from build123d import *

# Parameters (mm, degrees)
SKETCH2_W           = 52
SKETCH2_H           = 52
BOSS_EXTRUDE1_DEPTH = 70
SKETCH3_R           = 15
BOSS_EXTRUDE2_DEPTH = 20
SKETCH4_R           = 1
CUT_EXTRUDE1_DEPTH  = 5
SKETCH5_R           = 25
BOSS_EXTRUDE3_DEPTH = 8


with BuildPart() as part:
    # Sketch2 → Boss-Extrude1 (new body)
    with BuildSketch(Plane.XY):
        Rectangle(SKETCH2_W, SKETCH2_H)
    extrude(amount=BOSS_EXTRUDE1_DEPTH)

    # Sketch3 → Boss-Extrude2 (add)
    with BuildSketch(Plane.XY.offset(70)):
        Circle(SKETCH3_R)
    extrude(amount=BOSS_EXTRUDE2_DEPTH)

    # Sketch4 → Cut-Extrude1 (cut)
    with BuildSketch(Plane.XZ.offset(26)):
        with Locations((-16.5, 62)):
            Circle(SKETCH4_R)
        with Locations((-16.5, 28.5)):
            Circle(SKETCH4_R)
        with Locations((-1.5, 62)):
            Circle(SKETCH4_R)
        with Locations((-1.5, 28.5)):
            Circle(SKETCH4_R)
        with Locations((-1.5, 7)):
            Circle(SKETCH4_R)
        with Locations((-16.5, 7)):
            Circle(SKETCH4_R)
    extrude(amount=-CUT_EXTRUDE1_DEPTH, mode=Mode.SUBTRACT)

    # Sketch5 → Boss-Extrude3 (add)
    with BuildSketch(Plane.XY.offset(90)):
        Circle(SKETCH5_R)
    extrude(amount=-BOSS_EXTRUDE3_DEPTH)


solid = part.part
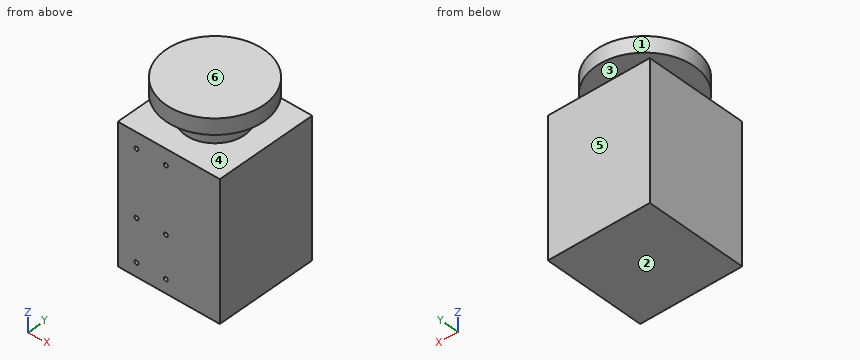
Verification items for the finished model (mm, model axes). Face numbers are marked on the shaded views. A direction names the side the tool comes from. Coordinates: 2 decimals unless noted, no trailing zeros. Order: outer loops, then holes, each group sorted by start corner. A loop starts at its lowest first (then second) coordinate and runs counter-clockwise, first axis right, second up.
Item 1: Section check D-D, the plane x = -1.5. Enter the section's corners in (y, z), then the cut area to 3 significant figures.
Filled in:
outline: (-26, 0) - (26, 0) - (26, 70) - (14.92, 70) - (14.92, 82) - (24.95, 82) - (24.95, 90) - (-24.95, 90) - (-24.95, 82) - (-14.92, 82) - (-14.92, 70) - (-26, 70) - (-26, 63) - (-21, 63) - (-21, 61) - (-26, 61) - (-26, 29.5) - (-21, 29.5) - (-21, 27.5) - (-26, 27.5) - (-26, 8) - (-21, 8) - (-21, 6) - (-26, 6) - close
area: 4,370 mm2
Item 2: Section check C-C, the plane y = -19.5. Enter the section's corners in (x, z).
Filled in:
outline: (-26, 0) - (26, 0) - (26, 70) - (-26, 70) - close; (-15.64, 82) - (15.64, 82) - (15.64, 90) - (-15.64, 90) - close
Item 3: Depth check by flat-ended pin: pin 1 (1.2 mm diameter, centred on x = -16.5, z = 28.5, fed in from -Y). Enter the tip coordinate at first touch or a pass-through.
Filled in:
pin 1: stops at y = -21
Item 4: Access from +Z, -Z, +X, -X, +Y, -Y to the whole of each face (thin tool, end or side, straight path). Record for the marked faces 1, 2 and 3.
Filled in:
face 1: +Z
face 2: -Z, +X, -X, +Y, -Y
face 3: none
Item 5: Material ranges on L1, parallel to Z at x = -1.5, y = -24; L2, parallel to Z at x = -21, y = 12.5; L3, parallel to Z at x = -16.5, y = -24, recorded low to high.
Filled in:
L1: z = 0 to 6, 8 to 27.5, 29.5 to 61, 63 to 70, 82 to 90
L2: z = 0 to 70, 82 to 90
L3: z = 0 to 6, 8 to 27.5, 29.5 to 61, 63 to 70
Item 6: Section check B-B, the plane y = 0. Enter the section's corners in (x, z).
Filled in:
outline: (-26, 0) - (26, 0) - (26, 70) - (15, 70) - (15, 82) - (25, 82) - (25, 90) - (-25, 90) - (-25, 82) - (-15, 82) - (-15, 70) - (-26, 70) - close
Item 7: Section check A-A, the plane x = -21. Enter the section's corners in (y, z).
Filled in:
outline: (-26, 0) - (26, 0) - (26, 70) - (-26, 70) - close; (-13.56, 82) - (13.56, 82) - (13.56, 90) - (-13.56, 90) - close
Item 8: Release check for a two-part mould opening along Z. For the marked faces 4, 5 and 6 record: +Z half, -Z half, draft (parallel to the pull), parting line (faces both ways), or undercut.
Filled in:
face 4: undercut
face 5: draft
face 6: +Z half
